Geometry check sheet. Reference: drawing and pictorial views, mm from the part's lowest x, y, z. Give positions to 0.01 mm unless a question says otherwise; leave off trailing zeros. Write each loop counter-clockwise with the first axis right and the second up, starting at its lowest first coordinate (ties: lowest second). Pieces come first, ordered by that corner, then holes. Notation, with made-up numbers: (13.25, 79.25) -> (27.25, 79.25) arc R24 ccw to (27.25, 104.25) -> close; hole circle Ø9 at (86.5, 17). An arc over 180 degrees is marked (long way). Answer as CSV lines item,"result".
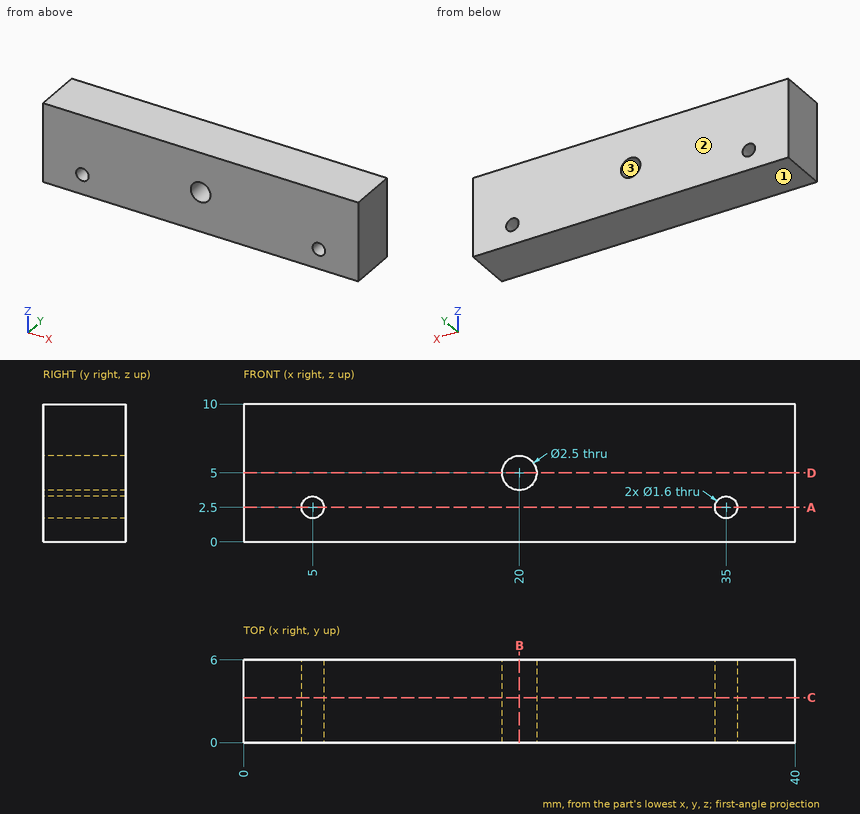
1) Draft check along Z on the marked faces 1, 2 and 3. Enter one of: +Z half, -Z half, draft (parallel to the pull), parting line (faces both ways), or undercut.
Reported:
face 1,"-Z half"
face 2,"draft"
face 3,"undercut"
2) Section check C-C (y = 3.25). Record the boundary of the cut face in (x, z), and give its area (3 significant figures).
Reported:
outline,"(0, 0) -> (40, 0) -> (40, 10) -> (0, 10) -> close; hole circle Ø1.6 at (5, 2.5); hole circle Ø2.5 at (20, 5); hole circle Ø1.6 at (35, 2.5)"
area,"391 mm²"
3) Depth check by flat-ended pin: pin 1 (1.3 mm diameter, centred on x = 5, z = 2.5, fed in from -Y). Enter the tip coordinate at first touch or a pass-through.
Reported:
pin 1,"through"
4) Section check A-A (z = 2.5). Record the boundary of the cut face in (x, y).
Reported:
outline,"(0, 0) -> (4.2, 0) -> (4.2, 6) -> (0, 6) -> close; (5.8, 0) -> (34.2, 0) -> (34.2, 6) -> (5.8, 6) -> close; (35.8, 0) -> (40, 0) -> (40, 6) -> (35.8, 6) -> close"
5) Section check D-D (z = 5). Record the boundary of the cut face in (x, y), and give its area (3 significant figures).
Reported:
outline,"(0, 0) -> (18.75, 0) -> (18.75, 6) -> (0, 6) -> close; (21.25, 0) -> (40, 0) -> (40, 6) -> (21.25, 6) -> close"
area,"225 mm²"
6) Section check B-B (x = 20). Record the boundary of the cut face in (y, z), and give its area (3 significant figures).
Reported:
outline,"(0, 0) -> (6, 0) -> (6, 3.75) -> (0, 3.75) -> close; (0, 6.25) -> (6, 6.25) -> (6, 10) -> (0, 10) -> close"
area,"45.0 mm²"
7) Scan lines: line 1 along X through (y, z) = (2.3, 3); line 2 along Z through (x, y) = (35, 2.1); line 3 along Z through (x, y) = (4.5, 5.4). Record each from-to range of solid material in increasing order.
Reported:
line 1,"0 to 4.38, 5.62 to 34.38, 35.62 to 40"
line 2,"0 to 1.7, 3.3 to 10"
line 3,"0 to 1.88, 3.12 to 10"
